```python
from build123d import *

# Parameters (mm, degrees)
ESQUISSE1_W                     = 85
ESQUISSE1_H                     = 70
BOSS_EXTRU_1_DEPTH              = 6
ESQUISSE3_R                     = 1.5
ENL_V_MAT_EXTRU_5_DEPTH         = 5
ESQUISSE5_R                     = 1.75
ENL_V_MAT_EXTRU_6_DEPTH         = 6
R_P_TITION_LIN_AIRE2_COUNT      = 6
R_P_TITION_LIN_AIRE2_PITCH      = 12
R_P_TITION_LIN_AIRE2_COUNT_DIR2 = 5
R_P_TITION_LIN_AIRE2_PITCH_DIR2 = 12
ESQUISSE8_R                     = 1.5
ENL_V_MAT_EXTRU_8_DEPTH         = 5
CUT_EXTRUDE2_DEPTH              = 56.38275905


with BuildPart() as part:
    # Esquisse1 → Boss.-Extru.1 (new body)
    with BuildSketch(Plane.XY):
        Rectangle(ESQUISSE1_W, ESQUISSE1_H)
    extrude(amount=BOSS_EXTRU_1_DEPTH)

    # Esquisse3 → Enlèv. mat.-Extru.5 (cut)
    with BuildSketch(Plane.ZY.offset(42.5)):
        with Locations((3, 0)):
            Circle(ESQUISSE3_R)
    enl_v_mat_extru_5 = extrude(amount=-ENL_V_MAT_EXTRU_5_DEPTH, mode=Mode.SUBTRACT)

    # Symétrie1: Enlèv. mat.-Extru.5 across plane
    add(enl_v_mat_extru_5.mirror(Plane(origin=(0, 0, 0), x_dir=(0, 0, 1), z_dir=(1, 0, 0))), mode=Mode.SUBTRACT)

    # Esquisse5 → Enlèv. mat.-Extru.6 (cut)
    with BuildSketch(Plane.XY):
        with Locations(Location((-31.5, -24, 0), (0, 0, 180))):
            Circle(ESQUISSE5_R)
    enl_v_mat_extru_6 = extrude(amount=ENL_V_MAT_EXTRU_6_DEPTH, mode=Mode.SUBTRACT)

    # Répétition linéaire2: Enl_v. mat.-Extru.6 6 × 5
    with Locations(*[(i * R_P_TITION_LIN_AIRE2_PITCH, j * R_P_TITION_LIN_AIRE2_PITCH_DIR2, 0) for i in range(R_P_TITION_LIN_AIRE2_COUNT) for j in range(R_P_TITION_LIN_AIRE2_COUNT_DIR2) if (i, j) != (0, 0)]):
        add(enl_v_mat_extru_6, mode=Mode.SUBTRACT)

    # Esquisse8 → Enlèv. mat.-Extru.8 (cut)
    with BuildSketch(Plane(origin=(0, 35, 0), x_dir=(1, 0, 0), z_dir=(0, 1, 0))):
        with Locations(Location((0, -3, 0), (0, 0, 270))):
            Circle(ESQUISSE8_R)
    enl_v_mat_extru_8 = extrude(amount=-ENL_V_MAT_EXTRU_8_DEPTH, mode=Mode.SUBTRACT)

    # Symétrie2: Enlèv. mat.-Extru.8 across plane
    add(enl_v_mat_extru_8.mirror(Plane.ZX), mode=Mode.SUBTRACT)

    # Sketch1 → Cut-Extrude2 (cut, through all)
    with BuildSketch(Plane(origin=(0, 0, 0), x_dir=(-1, 0, 0), z_dir=(0, 0, -1))):
        with BuildLine():
            Line((-2.5, -27), (-2.5, 28))
            ThreePointArc((-2.5, 28), (2.5, 33), (7.5, 28))
            Line((7.5, 28), (7.5, -27))
            ThreePointArc((7.5, -27), (2.5, -32), (-2.5, -27))
        make_face()
    extrude(amount=-CUT_EXTRUDE2_DEPTH, mode=Mode.SUBTRACT)


solid = part.part
```
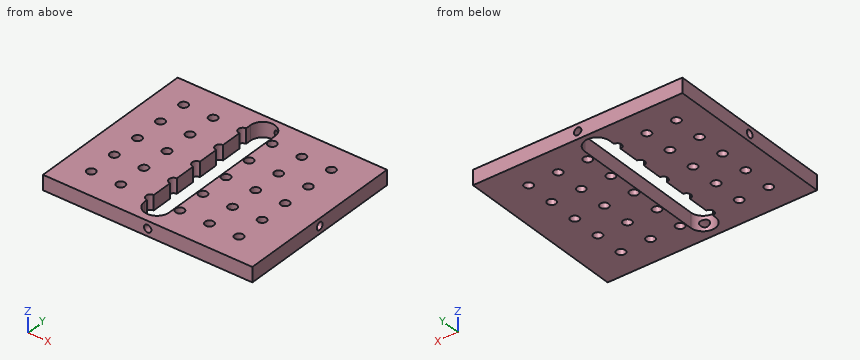
The model under review builds one solid part; all positions refer to its coordinate system, in mm. Give positions to 0.01 mm unless a question says otherwise; leave off trailing zeros. Write each loop counter-clockwise with the first axis right and the second up, starting at its lowest first coordinate (ties: lowest second). Pieces come first, ordered by that corner, then holes. Notation, with made-up numbers: M -28.5,77 L -6.5,77 A20 ccw -6.5,106 Z; hole C 8.5,-36.5 d9. An arc over 180 degrees is marked long. Write each question's results on one line, items separated by ' | '. Start each with the question number.
1. We need section C-C (x = -31.5). Write out the cut boundary in (y, z), and give its area (3 significant figures).
2. For probe 1 along Y at (x, z) = (-19.5, 3); probe 2 along X at (y, z) = (21, 0.75); probe 3 along Y at (x, z) = (15, 3), list the stretches that pass through material, from the lowest coordinate up. Write a range as [from, to].
3. Insertion check: pin 1 Ø0.9 at (y, z) = (0.5, 3.5) entering from +X; pin 2 Ø2 at (x, y) = (-19.5, -24) entering from -Z. Each pin has a flat end and moves straight along its axis. Give the tip position at first contact, or say it passes through.
4. We need section A-A (y = 7.5). Write out the cut boundary in (x, z), and give its area (3 significant figures).
5. We need section D-D (y = -12). Write out the cut boundary in (x, z).
6. We need section B-B (x = -2.5). Write out the cut boundary in (y, z), and give its area (3 significant figures).
Results found:
1) outline: M -35,0 L -25.75,0 L -25.75,6 L -35,6 Z; M -22.25,0 L -13.75,0 L -13.75,6 L -22.25,6 Z; M -10.25,0 L -1.75,0 L -1.75,6 L -10.25,6 Z; M 1.75,0 L 10.25,0 L 10.25,6 L 1.75,6 Z; M 13.75,0 L 22.25,0 L 22.25,6 L 13.75,6 Z; M 25.75,0 L 35,0 L 35,6 L 25.75,6 Z | area: 315 mm^2
2) probe 1: y = [-35, -25.75], [-22.25, -13.75], [-10.25, -1.75], [1.75, 10.25], [13.75, 22.25], [25.75, 35] | probe 2: x = [-42.5, -7.5], [2.5, 42.5] | probe 3: y = [-35, -24.9], [-23.1, -12.9], [-11.1, -0.9], [0.9, 11.1], [12.9, 23.1], [24.9, 35]
3) pin 1: stops at x = 37.5 | pin 2: passes through
4) outline: M -42.5,0 L -7.5,0 L -7.5,6 L -42.5,6 Z; M 2.5,0 L 42.5,0 L 42.5,6 L 2.5,6 Z | area: 450 mm^2
5) outline: M -42.5,0 L -33.25,0 L -33.25,6 L -42.5,6 Z; M -29.75,0 L -21.25,0 L -21.25,6 L -29.75,6 Z; M -17.75,0 L -9.25,0 L -9.25,6 L -17.75,6 Z; M 2.5,0 L 2.75,0 L 2.75,6 L 2.5,6 Z; M 6.25,0 L 14.75,0 L 14.75,6 L 6.25,6 Z; M 18.25,0 L 26.75,0 L 26.75,6 L 18.25,6 Z; M 30.25,0 L 42.5,0 L 42.5,6 L 30.25,6 Z
6) outline: M -35,0 L -32,0 L -32,6 L -35,6 Z; M 33,0 L 35,0 L 35,6 L 33,6 Z | area: 30.0 mm^2
